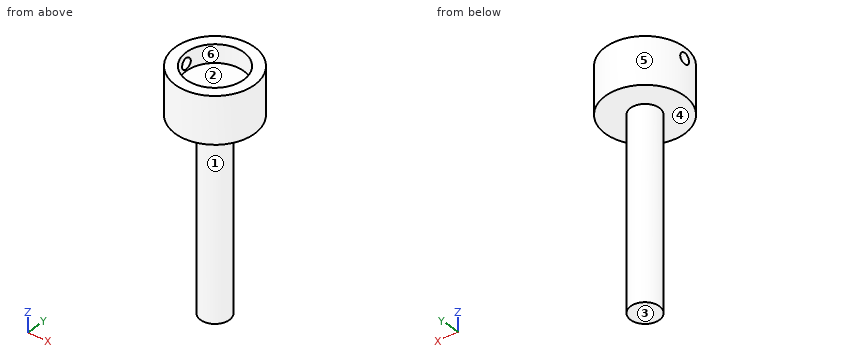
from build123d import *

# Parameters (mm, degrees)
CROQUIS1_R              = 11
SALIENTE_EXTRUIR1_DEPTH = 13
CROQUIS2_R              = 8
CORTAR_EXTRUIR1_DEPTH   = 5
CROQUIS3_R              = 1.5
CORTAR_EXTRUIR2_DEPTH   = 15
CROQUIS4_R              = 4
SALIENTE_EXTRUIR2_DEPTH = 52.8


with BuildPart() as part:
    # Croquis1 → Saliente-Extruir1 (new body)
    with BuildSketch(Plane.XY):
        Circle(CROQUIS1_R)
    extrude(amount=SALIENTE_EXTRUIR1_DEPTH)

    # Croquis2 → Cortar-Extruir1 (cut)
    with BuildSketch(Plane.XY.offset(13)):
        Circle(CROQUIS2_R)
    extrude(amount=-CORTAR_EXTRUIR1_DEPTH, mode=Mode.SUBTRACT)

    # Croquis3 → Cortar-Extruir2 (cut)
    with BuildSketch(Plane(origin=(0, 0, 0), x_dir=(0, 0, -1), z_dir=(1, 0, 0))):
        with Locations((-10, 0)):
            Circle(CROQUIS3_R)
    extrude(amount=-CORTAR_EXTRUIR2_DEPTH, mode=Mode.SUBTRACT)

    # Croquis4 → Saliente-Extruir2 (add)
    with BuildSketch(Plane(origin=(0, 0, 0), x_dir=(-1, 0, 0), z_dir=(0, 0, -1))):
        Circle(CROQUIS4_R)
    extrude(amount=SALIENTE_EXTRUIR2_DEPTH)


solid = part.part
Read the model definition and answer for the solid it produces. Units are mm, in the model's axes. Face numbers are marked on the shaded views. A direction names the side the tool comes from. Coordinates: 2 decimals unless noted, no trailing zeros. Order: outer loops, then holes, each group sorted by start corner. A loop starts at its lowest first (then second) coordinate and runs counter-clockwise, first axis right, second up. Notation, with made-up numbers: M -26,39.5 L -10,39.5 A4 cw -10,43.5 Z; hole C -23.75,5.5 d5. An arc over 180 degrees is marked long. Put each result on its own line as item: value. Start each with the question number.
Item 1: Section D-D, the plane y = 6.5 is taken. Determine the outline of the cut face in (x, z).
Item 2: For the marked faces 4, 5 and 6, determine the directions among +Z, -Z, +X, -X, +Y, -Y from which every point of the face is accessible in a straight line to the end or side of a thin tool.
Item 3: Given pin 1 Ø6 at (y, z) = (-3.5, 0.5) entering from +X; pin 2 Ø12 at (x, y) = (2.5, 6.5) entering from -Z; pin 3 Ø6 at (x, z) = (-5.5, -25) entering from -Y; pin 4 Ø3 at (x, y) = (5.5, -1) entering from +Z, each flat-ended and moving along its own axis, determine where each tip first touches the part or whether it passes through.
Item 4: Section A-A, the plane y = 0 is taken. Determine the outline of the cut face in (x, z).
Item 5: Section B-B, the plane x = 0 is taken. Determine the outline of the cut face in (y, z), plus the area to 3 significant figures.
Item 6: Section C-C, the plane z = -36 is taken. Determine the outline of the cut face in (x, y), plus the area to 3 significant figures.
Item 7: Consider probe 1 along Y at (x, z) = (0, 11.5); probe 2 along Z at (x, y) = (8.75, -0.5). Determine where each line is inside the solid, lowest interval first. Write a range as [from, to].
Item 8: The mould has two halves that part along X. Classify the marked faces 1, 2 and 3: +X half, -X half, draft (parallel to the pull), parting line (faces both ways), or undercut.
Computed:
1. outline: M -8.87,0 L 8.87,0 L 8.87,13 L 4.66,13 L 4.66,8 L -4.66,8 L -4.66,13 L -8.87,13 Z
2. face 4: -Z
2. face 5: +Z, -Z
2. face 6: +Z
3. pin 1: stops at x = 10.99
3. pin 2: stops at z = -52.8
3. pin 3: stops at y = -3.12
3. pin 4: stops at z = 8
4. outline: M -11,0 L -4,0 L -4,-52.8 L 4,-52.8 L 4,0 L 11,0 L 11,13 L 8,13 L 8,8 L -8,8 L -8,8.5 L -11,8.5 Z; M -11,11.5 L -8,11.5 L -8,13 L -11,13 Z
5. outline: M -11,0 L -4,0 L -4,-52.8 L 4,-52.8 L 4,0 L 11,0 L 11,13 L 8,13 L 8,8 L -8,8 L -8,13 L -11,13 Z
5. area: 628 mm2
6. outline: C 0,0 d8
6. area: 50.3 mm2
7. probe 1: y = [-11, -8], [8, 11]
7. probe 2: z = [0, 13]
8. face 1: parting line
8. face 2: undercut
8. face 3: draft
